```python
from build123d import *

# Parameters (mm, degrees)
SKETCH1_W                 = 27
SKETCH1_H                 = 22
BOSS_EXTRUDE1_DEPTH       = 12
SHELL1_T                  = -1.6
SKETCH2_W                 = 2
SKETCH2_H                 = 18.8
BOSS_EXTRUDE2_DEPTH       = 10.4
SKETCH4_R                 = 2
CUT_EXTRUDE2_DEPTH        = 9
SKETCH6_W                 = 10.34
SKETCH6_H                 = 12
BOSS_EXTRUDE4_DEPTH       = 5.5
SKETCH7_W                 = 25
SKETCH7_H                 = 5
BOSS_EXTRUDE5_DEPTH       = 5.25
CHAMFER1_SIZE             = 3
SKETCH8_R                 = 2
CUT_EXTRUDE3_DEPTH        = 33.994744773
CHAMFER2_SIZE             = 1.5
CHAMFER2_SIZE2            = 1.852345735
FILLET1_R                 = 2
CHAMFER1_OF_MIRROR1_SIZE  = 3
CHAMFER2_OF_MIRROR1_SIZE2 = 1.5
CHAMFER2_OF_MIRROR1_SIZE  = 1.852345735
FILLET1_OF_MIRROR1_R      = 2
BOSS_EXTRUDE7_START       = 1.2
BOSS_EXTRUDE7_DEPTH       = 1.2
SKETCH13_W                = 4.5
SKETCH13_H                = 22
CUT_EXTRUDE5_DEPTH        = 1
SKETCH17_W                = 11.66
SKETCH17_H                = 13.2
CUT_TOLERANCE_FIX_DEPTH   = 0.2
FILLET2_R                 = 1.5
SKETCH18_W                = 3.8
SKETCH18_H                = 5.9
BOSS_EXTRUDE8_DEPTH       = 10.4
SKETCH11_R                = 2
CUT_EXTRUDE6_DEPTH        = 10
SKETCH19_W                = 8
SKETCH19_H                = 18.8
BOSS_EXTRUDE9_DEPTH       = 2
SKETCH20_W                = 4.5
SKETCH20_H                = 22
CUT_EXTRUDE7_DEPTH        = 0.1
SKETCH21_W                = 7.8
SKETCH21_H                = 12.9
CUT_EXTRUDE8_DEPTH        = 2.05
CHAMFER4_SIZE             = 2
CHAMFER5_SIZE             = 3
TOLERANCE_ADJ_DEPTH       = 0.6
CHAMFER6_SIZE             = 0.5


with BuildPart() as part:
    # Sketch1 → Boss-Extrude1 (new body)
    with BuildSketch(Plane(origin=(0, 0, 0), x_dir=(1, 0, 0), z_dir=(0, 1, 0))):
        Rectangle(SKETCH1_W, SKETCH1_H)
    extrude(amount=BOSS_EXTRUDE1_DEPTH)

    # Shell1
    shell1_openings = [part.faces().sort_by_distance(p)[0] for p in [
        (0, 12, 0),
    ]]
    offset(amount=SHELL1_T, openings=shell1_openings, kind=Kind.INTERSECTION)

    # Sketch2 → Boss-Extrude2 (add)
    with BuildSketch(Plane(origin=(0, 1.6, 0), x_dir=(1, 0, 0), z_dir=(0, 1, 0))):
        with Locations((-2.9, 0)):
            Rectangle(SKETCH2_W, SKETCH2_H)
    boss_extrude2 = extrude(amount=BOSS_EXTRUDE2_DEPTH)

    # Sketch4 → Cut-Extrude2 (cut)
    with BuildSketch(Plane(origin=(0, 0, -11), x_dir=(-1, 0, 0), z_dir=(0, 0, -1))):
        with Locations((7.973688368, 6)):
            Circle(SKETCH4_R)
    cut_extrude2 = extrude(amount=-CUT_EXTRUDE2_DEPTH, mode=Mode.SUBTRACT)

    # Sketch6 → Boss-Extrude4 (add)
    with BuildSketch(Plane.ZY.offset(13.5)):
        with Locations((-5.83, 6)):
            Rectangle(SKETCH6_W, SKETCH6_H)
    boss_extrude4 = extrude(amount=BOSS_EXTRUDE4_DEPTH)

    # Sketch7 → Boss-Extrude5 (add)
    with BuildSketch(Plane.ZY.offset(19)):
        with Locations((6.383608836, 2.5)):
            Rectangle(SKETCH7_W, SKETCH7_H)
    boss_extrude5 = extrude(amount=BOSS_EXTRUDE5_DEPTH)

    # Chamfer1
    chamfer1_edges = [part.edges().sort_by_distance(p)[0] for p in [
        (-19, 2.5, -6.116391164),
    ]]
    chamfer(chamfer1_edges, length=CHAMFER1_SIZE)

    # Sketch8 → Cut-Extrude3 (cut, through all)
    with BuildSketch(Plane(origin=(0, 12, 0), x_dir=(1, 0, 0), z_dir=(0, 1, 0))):
        with Locations(Location((-15.5, 6, 0), (0, 0, 270))):
            Circle(SKETCH8_R)
    cut_extrude3 = extrude(amount=-CUT_EXTRUDE3_DEPTH, mode=Mode.SUBTRACT)

    # Chamfer2
    chamfer2_edges = [part.edges().sort_by_distance(p)[0] for p in [
        (-19, 2.5, -0.66),
    ]]
    chamfer2_side = [part.faces().sort_by_distance(p)[0] for p in [
        (-19, 2.5, 9.111804418),
    ]]
    chamfer(chamfer2_edges, length=CHAMFER2_SIZE, length2=CHAMFER2_SIZE2, reference=chamfer2_side[0])

    # Fillet1
    fillet1_edges = [part.edges().sort_by_distance(p)[0] for p in [
        (-19, 2.5, 18.883608836),
    ]]
    fillet(fillet1_edges, radius=FILLET1_R)

    # Mirror1: Boss-Extrude2, Cut-Extrude2, Boss-Extrude4, Boss-Extrude5, Cut-Extrude3 across plane
    add(boss_extrude2.mirror(Plane.ZY))
    add(cut_extrude2.mirror(Plane.ZY), mode=Mode.SUBTRACT)
    add(boss_extrude4.mirror(Plane.ZY))
    add(boss_extrude5.mirror(Plane.ZY))
    add(cut_extrude3.mirror(Plane.ZY), mode=Mode.SUBTRACT)

    # Chamfer1 of Mirror1
    chamfer1_of_mirror1_edges = [part.edges().sort_by_distance(p)[0] for p in [
        (19, 2.5, -6.116391164),
    ]]
    chamfer(chamfer1_of_mirror1_edges, length=CHAMFER1_OF_MIRROR1_SIZE)

    # Chamfer2 of Mirror1
    chamfer2_of_mirror1_edges = [part.edges().sort_by_distance(p)[0] for p in [
        (19, 2.5, -0.66),
    ]]
    chamfer(chamfer2_of_mirror1_edges, length=CHAMFER2_OF_MIRROR1_SIZE, length2=CHAMFER2_OF_MIRROR1_SIZE2)

    # Fillet1 of Mirror1
    fillet1_of_mirror1_edges = [part.edges().sort_by_distance(p)[0] for p in [
        (19, 2.5, 18.883608836),
    ]]
    fillet(fillet1_of_mirror1_edges, radius=FILLET1_OF_MIRROR1_R)

    # Sketch12 → Boss-Extrude7 (add)
    with BuildSketch(Plane.XZ.offset(BOSS_EXTRUDE7_START)):
        with BuildLine():
            Line((6.6, 11), (-13.5, 11))
            Line((-13.5, 11), (-13.5, -0.66))
            Line((-13.5, -0.66), (-17.147654265, -0.66))
            Line((-17.147654265, -0.66), (-19, 0.84))
            Line((-19, 0.84), (-19, 16.883608836))
            ThreePointArc((-19, 16.883608836), (-19.585786438, 18.297822398), (-21, 18.883608836))
            Line((-21, 18.883608836), (-24.25, 18.883608836))
            Line((-24.25, 18.883608836), (-24.25, -6.116391164))
            Line((-24.25, -6.116391164), (-22, -6.116391164))
            Line((-22, -6.116391164), (-19, -9.116391164))
            Line((-19, -9.116391164), (-19, -11))
            Line((-19, -11), (6.6, -11))
            Line((6.6, -11), (6.6, 11))
        make_face()
        with BuildLine():
            Line((11.1, -11), (11.1, 11))
            Line((11.1, 11), (13.5, 11))
            Line((13.5, 11), (13.5, -0.66))
            Line((13.5, -0.66), (17.147654265, -0.66))
            Line((17.147654265, -0.66), (19, 0.84))
            Line((19, 0.84), (19, 16.883608836))
            ThreePointArc((19, 16.883608836), (19.585786438, 18.297822398), (21, 18.883608836))
            Line((21, 18.883608836), (24.25, 18.883608836))
            Line((24.25, 18.883608836), (24.25, -6.116391164))
            Line((24.25, -6.116391164), (22, -6.116391164))
            Line((22, -6.116391164), (19, -9.116391164))
            Line((19, -9.116391164), (19, -11))
            Line((19, -11), (11.1, -11))
        make_face()
    extrude(amount=-BOSS_EXTRUDE7_DEPTH)

    # Sketch13 → Cut-Extrude5 (cut)
    with BuildSketch(Plane(origin=(0, 0, 0), x_dir=(-1, 0, 0), z_dir=(0, -1, 0))):
        with Locations((-8.85, 0)):
            Rectangle(SKETCH13_W, SKETCH13_H)
    extrude(amount=-CUT_EXTRUDE5_DEPTH, mode=Mode.SUBTRACT)

    # Sketch17 → Cut- tolerance fix (cut)
    with BuildSketch(Plane.ZY.offset(13.5)):
        with Locations((5.17, 5.4)):
            Rectangle(SKETCH17_W, SKETCH17_H)
    cut_tolerance_fix = extrude(amount=-CUT_TOLERANCE_FIX_DEPTH, mode=Mode.SUBTRACT)

    # Mirror2: Cut- tolerance fix across plane
    add(cut_tolerance_fix.mirror(Plane.ZY), mode=Mode.SUBTRACT)

    # Fillet2
    fillet2_edges = [part.edges().sort_by_distance(p)[0] for p in [
        (-3.35, -1.2, 11),
        (12.2, -1.2, 11),
    ]]
    fillet(fillet2_edges, radius=FILLET2_R)

    # Sketch18 → Boss-Extrude8 (add)
    with BuildSketch(Plane(origin=(0, 1.6, 0), x_dir=(1, 0, 0), z_dir=(0, 1, 0))):
        with Locations((0, -6.45)):
            Rectangle(SKETCH18_W, SKETCH18_H)
    extrude(amount=BOSS_EXTRUDE8_DEPTH)

    # Sketch11 → Cut-Extrude6 (cut)
    with BuildSketch(Plane(origin=(0, 12, 0), x_dir=(1, 0, 0), z_dir=(0, 1, 0))):
        with Locations(Location((0, -7.181115317, 0), (0, 0, 270))):
            Circle(SKETCH11_R)
    extrude(amount=-CUT_EXTRUDE6_DEPTH, mode=Mode.SUBTRACT)

    # Sketch19 → Boss-Extrude9 (add)
    with BuildSketch(Plane(origin=(0, 1.6, 0), x_dir=(1, 0, 0), z_dir=(0, 1, 0))):
        with Locations((7.9, 0)):
            Rectangle(SKETCH19_W, SKETCH19_H)
        with Locations((-7.9, 0)):
            Rectangle(SKETCH19_W, SKETCH19_H)
    extrude(amount=BOSS_EXTRUDE9_DEPTH)

    # Sketch20 → Cut-Extrude7 (cut)
    with BuildSketch(Plane.XZ.offset(-1)):
        with Locations((8.85, 0)):
            Rectangle(SKETCH20_W, SKETCH20_H)
    extrude(amount=-CUT_EXTRUDE7_DEPTH, mode=Mode.SUBTRACT)

    # Sketch21 → Cut-Extrude8 (cut)
    with BuildSketch(Plane(origin=(0, 12, 0), x_dir=(1, 0, 0), z_dir=(0, 1, 0))):
        with Locations((0, 2.95)):
            Rectangle(SKETCH21_W, SKETCH21_H)
    extrude(amount=-CUT_EXTRUDE8_DEPTH, mode=Mode.SUBTRACT)

    # Chamfer4
    chamfer4_edges = [part.edges().sort_by_distance(p)[0] for p in [
        (-2.9, 9.95, -9.4),
        (-2.9, 9.95, 3.5),
        (2.9, 9.95, -9.4),
        (2.9, 9.95, 3.5),
    ]]
    chamfer(chamfer4_edges, length=CHAMFER4_SIZE)

    # Chamfer5
    chamfer5_edges = [part.edges().sort_by_distance(p)[0] for p in [
        (-18.073827133, 5, -0.66),
        (-19, 5, -4.888195582),
        (18.073827133, 5, -0.66),
        (19, 5, -4.888195582),
    ]]
    chamfer(chamfer5_edges, length=CHAMFER5_SIZE)

    # Sketch22 → tolerance adj (cut)
    with BuildSketch(Plane(origin=(6.6, 0, 0), x_dir=(0, 0, -1), z_dir=(1, 0, 0))):
        with BuildLine():
            Line((-11, 1.1), (-11, 0.3))
            ThreePointArc((-11, 0.3), (-10.560660172, -0.760660172), (-9.5, -1.2))
            Line((-9.5, -1.2), (11, -1.2))
            Line((11, -1.2), (11, 1.1))
            Line((11, 1.1), (-11, 1.1))
        make_face()
    extrude(amount=-TOLERANCE_ADJ_DEPTH, mode=Mode.SUBTRACT)

    # Chamfer6
    chamfer6_edges = [part.edges().sort_by_distance(p)[0] for p in [
        (-13.3, -1.2, 4.42),
        (13.3, -1.2, 4.42),
        (11.1, -1.2, -0.75),
        (11.1, 0.7, 11),
        (11.1, -0.760660172, 10.560660172),
        (13.3, 6.15, 11),
        (-13.3, 6.15, 11),
        (13.3, -0.760660172, 10.560660172),
        (-13.3, -0.760660172, 10.560660172),
        (6, -1.2, -0.75),
        (6, -0.760660172, 10.560660172),
        (6, 0.7, 11),
    ]]
    chamfer(chamfer6_edges, length=CHAMFER6_SIZE)


solid = part.part
```
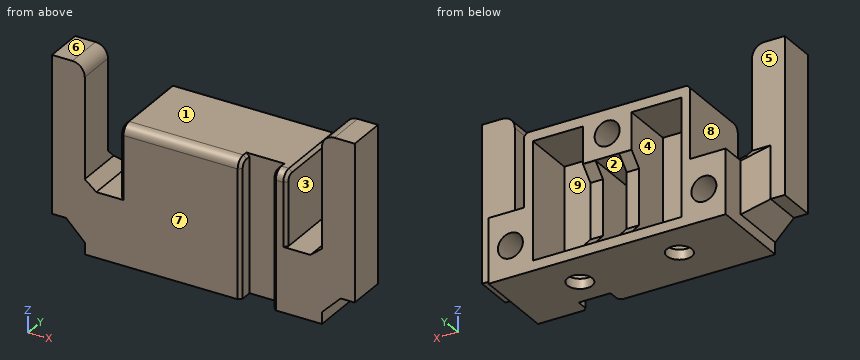
Work out the finished part from the listing and answer in its coordinate system (mm). Face numbers are marked on the shaded views. A direction names the side the tool comes from. Round coordinates to 2 decimals unless told otherwise and drop trailing zeros. Loops run counter-clockwise (first coordinate to the right, second up) from the corner with the lowest first, then second, coordinate; pieces in that order, holes last. Notation, with made-up numbers: M 57.25,20 L 97.25,20 A16 cw 97.25,47 Z; hole C -0.5,70.5 d4. An arc over 180 degrees is marked long. Use CSV: the item, a comma, the result in double quotes.
Q1. Each of these flat-tipped pins is pushed along its axis until it touches: pin 1 (1.2 mm diameter, centred on x = -0.5, z = 7, fed in from +Y); pin 2 (2 mm diameter, centred on x = 4.5, y = 4, fed in from +Z); pin 3 (3 mm diameter, centred on x = 16.5, y = 8.5, fed in from +Z). Where does it stop, or does it pass through?
Determined:
pin 1,"y = 2"
pin 2,"z = 11"
pin 3,"z = -0.23"
Q2. Section C-C, the plane z = 6.5 is taken. State how many separate pieces and enclosed holes the cut face has, then the cut area to 3 significant figures.
Determined:
separate pieces,"3"
enclosed holes,"0"
area,"232 mm2"
Q3. Section D-D, the plane x = -9 is taken. Determine the outline of the cut face in (y, z).
Determined:
outline,"M -1.2,-11 L 4.28,-11 L 4.28,-9.4 L 3.6,-9.4 L 3.6,9.4 L 12,9.4 L 12,11 L 0.3,11 A1.5 ccw -1.2,9.5 Z; M 7.72,-11 L 12,-11 L 12,-9.4 L 7.72,-9.4 Z"
Q4. A tool of negligible diameter and unlimited length cuts with its end or side. For the marked faces 5, 6, 7, 8 and 9, from which of +Z, -Z, +X, -X, +Y, -Y can it reach the whole face along a straight path? Write none if from no direction.
Determined:
face 5,"+Z, -X, +Y"
face 6,"+Z, +X, -X, +Y, -Y"
face 7,"+Z, -Z, +X, -X, -Y"
face 8,"+Z, +Y, -Y"
face 9,"+Y"
Q5. Consider L1, parallel to X at y = 10, z = 2; L2, parallel to X at y = 0.5, z = 11.25; L3, parallel to X at y = 11.5, z = 1.75. Determine where each line is inside the solid, lowest interval first.
Determined:
L1,"-13.3 to -11.9, -3.9 to -1.9, 1.9 to 3.9, 11.9 to 13.3"
L2,"-24.25 to -19, 19 to 24.25"
L3,"-13.3 to -11.9, 11.9 to 13.3"
Q6. Section A-A, the plane z = 11.75 is taken. Determine the outline of the cut face in (x, y), then the cut area to 3 significant figures.
Determined:
outline,"M -24.25,-1.2 L -19,-1.2 L -19,5 L -24.25,5 Z; M 19,-1.2 L 24.25,-1.2 L 24.25,5 L 19,5 Z"
area,"65.1 mm2"
Q7. The mould has two halves that part along Z. Classify the marked faces 1, 2, 3 and 4: pulls with the +Z half, pulls with the -Z half, needs draft (parallel to the pull), parting line crosses it, or undercut.
Determined:
face 1,"pulls with the +Z half"
face 2,"undercut"
face 3,"needs draft"
face 4,"undercut"
Q8. Section B-B, the plane x = 0 is taken. Determine the outline of the cut face in (y, z), then the cut area to 3 significant figures.
Determined:
outline,"M -1.2,-11 L 12,-11 L 12,-9.4 L 1.6,-9.4 L 1.6,3.5 L 12,3.5 L 12,5.18 L 2,5.18 L 2,9.18 L 12,9.18 L 12,11 L 0.3,11 A1.5 ccw -1.2,9.5 Z"
area,"116 mm2"
